Autodesk Inventor part; units mm, degrees
ref_plane "YZ Plane" through (0, 0, 0) normal (1, 0, 0) x (0, 1, 0)
ref_plane "XZ Plane" through (0, 0, 0) normal (0, 1, 0) x (-1, 0, 0)
ref_plane "XY Plane" through (0, 0, 0) normal (0, 0, 1) x (1, 0, 0)
sketch "Szkic1" plane through (0, 0, 0) normal (0, 0, 1) x (1, 0, 0)
  line L0 (0, 0) -> (55, 0)
  line L1 (55, 0) -> (55, 65)
  line L2 (55, 65) -> (0, 65)
  line L3 (0, 65) -> (0, 0)
  dimension "d0" = 55
  dimension "d1" = 65
extrude "Wyciągnięcie proste1" add sketch "Szkic1" along normal blind 1.6
sketch "Szkic2" plane through (0, 0, 1.6) normal (0, 0, 1) x (1, 0, 0)
  circle A0 centre (50, 35) radius 0.6
  circle A1 centre (45, 35) radius 0.6
  circle A2 centre (40, 35) radius 0.6
  circle A3 centre (32.5, 20) radius 0.6
  circle A4 centre (27.5, 20) radius 0.6
  circle A5 centre (22.5, 20) radius 0.6
  circle A6 centre (15, 35) radius 0.6
  circle A7 centre (10, 35) radius 0.6
  circle A8 centre (5, 35) radius 0.6
  line L0 (55, 65) -> (0, 65)
  point P0 (0, 0)
  point P1 (27.5, 65)
  dimension "d4" = 15
  dimension "d5" = 5
  dimension "d6" = 5
  dimension "d7" = 5
  dimension "d8" = 5
  dimension "d9" = 5
  dimension "d10" = 5
  dimension "d11" = 30
  dimension "d12" = 17.5
  dimension "d13" = 17.5
  dimension "d14" = 1.2
extrude "Wyciągnięcie proste2" cut sketch "Szkic2" against normal blind 1.6
sketch "Szkic3" plane through (0, 0, 1.6) normal (0, 0, 1) x (1, 0, 0)
  circle A0 centre (27.5, 53.25) radius 4
  point P0 (0, 0)
extrude "Wyciągnięcie proste3" cut sketch "Szkic3" against normal blind 1.6
equation "\"d6\" = d5"
equation "\"d7\" = d6"
equation "\"d8\" = d7"
equation "\"d9\" = d8"
equation "\"d10\" = d9"
equation "\"d13\" = d12"
properties part number "pcb main"
Source: CAD feature listing. Evaluate the final solid. Frame: model axes, mm. Round coordinates to 2 decimals unless told otherwise and drop trailing zeros. Loops run counter-clockwise (first coordinate to the right, second up) from the corner with the lowest first, then second, coordinate; pieces in that order, holes last. Notation, with made-up numbers: M 72.5,86.25 L 91.5,86.25 A14 ccw 91.5,95.25 Z; hole C -31,-8 d11. An arc over 180 degrees is marked long. Use a Markdown table: item, result. Add a question column.
1. Line query: line 1 (Y direction, x = 27.5, z = 0.6); line 2 (Y direction, x = 32.5, z = 0.9); line 3 (X direction, y = 53.5, z = 0.95). Output: solid intervals per line, ascending.
2. Mould query, pull axis X, two halves, no side actions, for faces 1 (the flat face through (27, 33, 0)), 2 (the flat face through (0, 33, 1)), 3 (the cylindrical face through (26.633, 49.345, 0.811)). Classes: pulls with the +X half, pulls with the -X half, needs draft (parallel to the pull), parting line crosses it, or undercut.
3. Contact query for flat-ended pins moving along their axis: P1, Ø1, axis at x = 15, y = 35, coming from the +Z side; P2, Ø1.4, axis at x = 22.5, y = 20, coming from the -Z side. Output: stop coordinate, or through.
4. Section query A-A on z = 0.6. Give the number of separate pieces and of enclosed holes in the cut face, then the cut area to 3 significant figures.
5. Section query B-B on y = 55.5. Return the cut outline in (x, z), then the cut area to 3 significant figures.
Reported:
| question | item | result |
|---|---|---|
| 1 | line 1 | y = 0 to 19.4, 20.6 to 49.25, 57.25 to 65 |
| 1 | line 2 | y = 0 to 19.4, 20.6 to 65 |
| 1 | line 3 | x = 0 to 23.51, 31.49 to 55 |
| 2 | face 1 | needs draft |
| 2 | face 2 | pulls with the -X half |
| 2 | face 3 | undercut |
| 3 | P1 | passes through |
| 3 | P2 | stops at z = 0 |
| 4 | separate pieces | 1 |
| 4 | enclosed holes | 10 |
| 4 | area | 3,510 mm² |
| 5 | outline | M 0,0 L 24.19,0 L 24.19,1.6 L 0,1.6 Z; M 30.81,0 L 55,0 L 55,1.6 L 30.81,1.6 Z |
| 5 | area | 77.4 mm² |
